The figure shows three views and two pictorial views of one solid part (mm, origin at its lowest corner). Answer the questions. A direction names the side the tool comes from. Coordinates: 2 decimals unless noted, no trailing zeros. Write each loop counter-clockwise with the first axis right and the second up, starting at its lowest first coordinate (ties: lowest second). Pieces come first, ordered by that corner, then holes. Notation, with made-up numbers: (46.25, 24.25) -> (62.25, 24.25) arc R35 cw to (62.25, 57.25) -> close; hole circle Ø5 at (-12, 19.5). An arc over 180 degrees is marked (long way). Use CSV: the item, a comma, the result in double quotes. Start each with the question number.
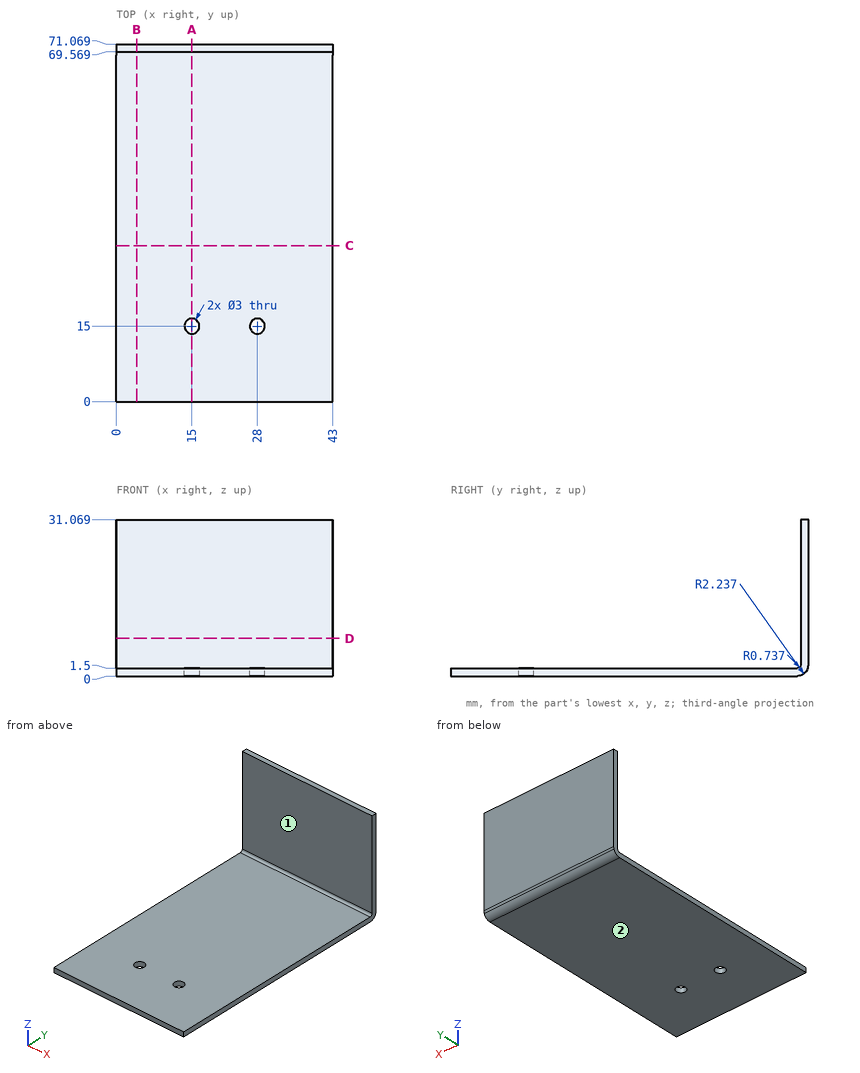
1) Section D-D, the plane z = 7.5 is taken. Give the vertices of the cut face in (x, y).
2) Which of the six approach directions +Z, -Z, +X, -X, +Y, -Y give full straight-line access (tool end or side, diameter ignored) to the marked faces 1 and 2?
3) Find the intervals of material crossed by line 1 along X through (y, z) = (15, 0.6); line 2 along Y through (x, z) = (34, 10); line 3 along Z through (x, y) = (32.5, 63.5), in increasing order.
4) Section B-B, the plane x = 4 is taken. Give the vertices of the cut face in (y, z) (1 decimal).
5) Section A-A, the plane x = 15 is taken. Give the vertices of the cut face in (y, z) (1 decimal).
6) Section C-C, the plane y = 31 is taken. Give the vertices of the cut face in (x, z).
7) Each of these flat-tipped pins is pushed along its axis until it touches: pin 1 (1.5 mm diameter, centred on x = 25.5, y = 30, fed in from +Z); pin 2 (1.5 mm diameter, centred on x = 13.5, z = 11, fed in from -Y). Where does it stop, or does it pass through?
The answers:
1,outline,"(0, 69.57) -> (43, 69.57) -> (43, 71.07) -> (0, 71.07) -> close"
2,face 1,"+Z, +X, -X, -Y"
2,face 2,"-Z, +X, -X, +Y, -Y"
3,line 1,"x = 0 to 13.5, 16.5 to 26.5, 29.5 to 43"
3,line 2,"y = 69.57 to 71.07"
3,line 3,"z = 0 to 1.5"
4,outline,"(0, 0) -> (68.8, 0) arc R2.2 ccw to (71.1, 2.2) -> (71.1, 31.1) -> (69.6, 31.1) -> (69.6, 2.2) arc R0.7 cw to (68.8, 1.5) -> (0, 1.5) -> close"
5,outline,"(0, 0) -> (13.5, 0) -> (13.5, 1.5) -> (0, 1.5) -> close; (16.5, 0) -> (68.8, 0) arc R2.2 ccw to (71.1, 2.2) -> (71.1, 31.1) -> (69.6, 31.1) -> (69.6, 2.2) arc R0.7 cw to (68.8, 1.5) -> (16.5, 1.5) -> close"
6,outline,"(0, 0) -> (43, 0) -> (43, 1.5) -> (0, 1.5) -> close"
7,pin 1,"stops at z = 1.5"
7,pin 2,"stops at y = 69.57"
